```python
from build123d import *

# Parameters (mm, degrees)
F0_W     = 110
F0_H     = 80
F1_DEPTH = 10
F3_DEPTH = 100
F4_R     = 4


with BuildPart() as f1:
    # F0 (on Top) → F1 (new body)
    with BuildSketch(Plane.XY):
        with Locations((55, 40)):
            Rectangle(F0_W, F0_H)
    extrude(amount=F1_DEPTH)

    # F2 (on face) → F3 (cut)
    with BuildSketch(Plane(origin=(0, 0, 0), x_dir=(0, -1, 0), z_dir=(-1, 0, 0))):
        Polygon((-53, 10), (-60, 10), (-62.5, 2.4006579232), (-50.5, 2.4006579232), align=None)
        Polygon((-20, 10), (-27, 10), (-29.5, 2.4006579232), (-17.5, 2.4006579232), align=None)
    extrude(amount=-F3_DEPTH, mode=Mode.SUBTRACT)

    # F4
    f4_edges = [f1.edges().sort_by_distance(p)[0] for p in [
        (0, 0, 5),
        (110, 0, 5),
        (110, 80, 5),
        (0, 80, 5),
        (55, 80, 10),
        (110, 40, 10),
        (55, 0, 10),
        (0, 10, 10),
        (0, 40, 10),
        (0, 70, 10),
    ]]
    fillet(f4_edges, radius=F4_R)


solid = f1.part
```
Source: CAD feature listing. Evaluate the final solid. Frame: model axes, mm. A direction names the side the tool comes from. Coordinates: 2 decimals unless noted, no trailing zeros. Write each loop counter-clockwise with the first axis right and the second up, starting at its lowest first coordinate (ties: lowest second). Pieces come first, ordered by that corner, then holes. Notation, with made-up numbers: (-31, 83.25) - (14, 83.25) arc R28 ccw to (14, 106.25) - close; hole circle Ø8 at (-13, 29). An arc over 180 degrees is marked (long way). Answer as a JSON object with one key per item and string values.
Q1. Material intervals for line 1 (Y direction, x = 23, z = 5); line 2 (Y direction, x = 79.5, z = 7.5); line 3 (X direction, y = 28, z = 8.75), sorted ascending. Write a range as [from, to].
Ans:
{"line 1": "y = [0, 18.36], [28.64, 51.36], [61.64, 80]", "line 2": "y = [0.29, 19.18], [27.82, 52.18], [60.82, 79.71]", "line 3": "x = [1.1, 108.9]"}
Q2. Draft query along Y for faces 1 (the flat face through (54, 0, 3)), 2 (the flat face through (54, 80, 3)), 3 (the cylindrical face through (1.141, 12.112, 8.797)), 4 (the flat face through (49, 57, 2.401)). Return one class per face: released by +Y, released by -Y, zero draft, split by the parting line, or undercut.
Ans:
{"face 1": "released by -Y", "face 2": "released by +Y", "face 3": "zero draft", "face 4": "undercut"}
Q3. Section query A-A, the plane x = 26.5. Output: boundary loops of the cut face in (y, z).
Ans:
{"outline": "(0, 0) - (80, 0) - (80, 6) arc R4 ccw to (76, 10) - (60, 10) - (62.5, 2.4) - (50.5, 2.4) - (53, 10) - (27, 10) - (29.5, 2.4) - (17.5, 2.4) - (20, 10) - (4, 10) arc R4 ccw to (0, 6) - close"}
Q4. First-contact query: pin 1 Ø3 at (y, z) = (55, 5.5) entering from -X; pin 2 Ø6 at (y, z) = (58, 8) entering from -X. Flat tips, straight axial feed; report the tip coordinate or a pass-through.
Ans:
{"pin 1": "stops at x = 100", "pin 2": "stops at x = 0.2"}
Q5. Section query B-B, the plane z = 7.25. Output: boundary loops of the cut face in (x, y), plus the area to 3 significant figures.
Ans:
{"outline": "(0.2, 4) arc R3.8 ccw to (4, 0.2) - (106, 0.2) arc R3.8 ccw to (109.8, 4) - (109.8, 76) arc R3.8 ccw to (106, 79.8) - (4, 79.8) arc R3.8 ccw to (0.2, 76) - (0.2, 60.9) - (100, 60.9) - (100, 52.1) - (0.2, 52.1) - (0.2, 27.9) - (100, 27.9) - (100, 19.1) - (0.2, 19.1) - close", "area": "6,950 mm2"}
Q6. Set-up query: faces 5 (the flat face through (49.3, 28.232, 6.254)), 6 (the flat face through (0, 39, 3)). Return all of +Z, -Z, +X, -X, +Y, -Y with unobstructed straight access to the full face (end or side cutting, diameter ignored); none if empty.
Ans:
{"face 5": "-X", "face 6": "+Z, -Z, -X, +Y, -Y"}
